Work out the finished part from the listing and answer in its coordinate system (mm). Face numbers are marked on the shaded views. A direction names the side the tool comes from. Coordinates: 2 decimals unless noted, no trailing zeros. Write each loop counter-clockwise with the first axis right and the second up, starting at its lowest first coordinate (ties: lowest second). Pieces come first, ordered by that corner, then holes. Notation, with made-up numbers: M -18,-19.5 L -7,-19.5 A13 ccw -7,-11.5 Z; hole C 70,28.5 d5. An arc over 180 degrees is marked long. Use CSV: the item, a comma, the result in double quotes.
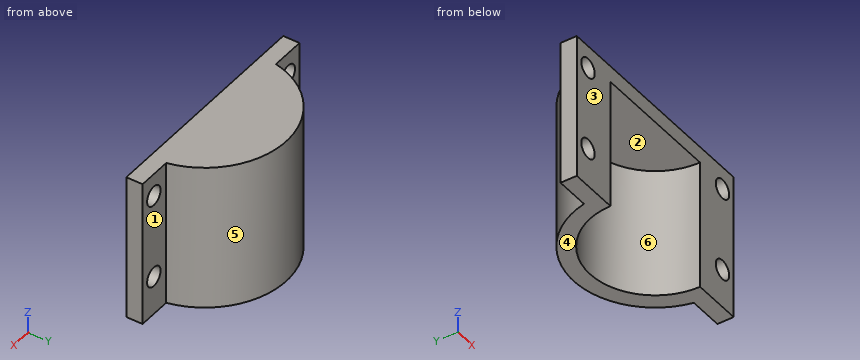
from build123d import *

# Parameters (mm, degrees)
SKETCH1_W                 = 70
SKETCH1_H                 = 50
BOSS_EXTRUDE1_DEPTH       = 30
CAVITY1_START             = -20
CAVITY1_DEPTH             = 40
CAVITY1_START_2           = -25
CAVITY1_2_DEPTH           = 5
CUT_EXTRUDE1_DEPTH        = 65.420493634
CUT_EXTRUDE1_DEPTH_BACK   = 65.420493634
F_6_0MM_DOWEL_HOLE1_D     = 6
F_6_0MM_DOWEL_HOLE1_DEPTH = 10
F_6_0MM_DOWEL_HOLE1_TIP   = 1.802581857
CUT_EXTRUDE3_DEPTH        = 5


# Read off the part's stored shape, not the designer's step: Cavity1
with BuildPart() as part:
    # Sketch1 → Boss-Extrude1 (new body)
    with BuildSketch(Plane(origin=(0, 0, 0), x_dir=(1, 0, 0), z_dir=(0, 1, 0))):
        Rectangle(SKETCH1_W, SKETCH1_H)
    extrude(amount=BOSS_EXTRUDE1_DEPTH)

    # Cavity1 outline → Cavity1 (cut)
    with BuildSketch(Plane.XY.offset(CAVITY1_START)):
        with BuildLine():
            ThreePointArc((20, 0), (0, 20), (-20, 0))
            Line((-20, 0), (20, 0))
        make_face()
    extrude(amount=CAVITY1_DEPTH, mode=Mode.SUBTRACT)

    # Cavity1 2 outline → Cavity1 2 (cut)
    with BuildSketch(Plane.XY.offset(CAVITY1_START_2)):
        with BuildLine():
            Line((-10, 0), (10, 0))
            ThreePointArc((10, 0), (0, 10), (-10, 0))
        make_face()
    extrude(amount=CAVITY1_2_DEPTH, mode=Mode.SUBTRACT)

    # Sketch2 → Cut-Extrude1 (cut, two sides: drawn at the far end of the back side and taken through both)
    with BuildSketch(Plane(origin=(0, 0, 20), x_dir=(-1, 0, 0), z_dir=(0, 0, -1)).offset(-CUT_EXTRUDE1_DEPTH_BACK)):
        with BuildLine():
            Line((-35, 30), (-35, 5))
            Line((-35, 5), (-24.494897428, 5))
            ThreePointArc((-24.494897428, 5), (0, 25), (24.494897428, 5))
            Line((24.494897428, 5), (35, 5))
            Line((35, 5), (35, 30))
            Line((35, 30), (-35, 30))
        make_face()
    extrude(amount=CUT_EXTRUDE1_DEPTH + CUT_EXTRUDE1_DEPTH_BACK, mode=Mode.SUBTRACT)

    # Ø6.0mm Dowel Hole1
    with Locations(Plane(origin=(0, 0, 0), x_dir=(-1, 0, 0), z_dir=(0, -1, 0))):
        with Locations((-30, 8), (-30, -18), (30, 8), (30, -18)):
            Hole(F_6_0MM_DOWEL_HOLE1_D / 2, depth=F_6_0MM_DOWEL_HOLE1_DEPTH)
            with Locations((0, 0, -(F_6_0MM_DOWEL_HOLE1_DEPTH + F_6_0MM_DOWEL_HOLE1_TIP / 2))):  # 118° drill point
                Cone(0, F_6_0MM_DOWEL_HOLE1_D / 2, F_6_0MM_DOWEL_HOLE1_TIP, mode=Mode.SUBTRACT)

    # Sketch6 → Cut-Extrude3 (cut)
    with BuildSketch(Plane(origin=(0, 0, -25), x_dir=(-1, 0, 0), z_dir=(0, 0, -1))):
        with BuildLine():
            Line((35, 5), (24.494897428, 5))
            ThreePointArc((24.494897428, 5), (0, 25), (-24.494897428, 5))
            Line((-24.494897428, 5), (-35, 5))
            Line((-35, 5), (-35, 0))
            Line((-35, 0), (-10, 0))
            ThreePointArc((-10, 0), (0, 10), (10, 0))
            Line((10, 0), (35, 0))
            Line((35, 0), (35, 5))
        make_face()
    extrude(amount=-CUT_EXTRUDE3_DEPTH, mode=Mode.SUBTRACT)


solid = part.part
Item 1: A tool of negligible diameter and unlimited length cuts with its end or side. For the marked faces 1, 2 and 3, from which of +Z, -Z, +X, -X, +Y, -Y can it reach the whole face along a straight path? Write none if from no direction.
Answer:
face 1,"+Z, -Z, +X, +Y"
face 2,"-Z, -Y"
face 3,"+Z, -Z, +X, -X, -Y"
Item 2: The part is cut by section A-A (x = -30). Write down the section's boundary in (y, z), then the cut area to 3 significant figures.
Answer:
outline,"M 0,-20 L 5,-20 L 5,-11 L 0,-11 Z; M 0,-5 L 5,-5 L 5,15 L 0,15 Z; M 0,21 L 5,21 L 5,25 L 0,25 Z"
area,"165 mm2"
Item 3: For a pull along X with two mould halves and no side action, classify the marked faces 4, 5 and 6 as released by +X, released by -X, zero draft, split by the parting line, or undercut.
Answer:
face 4,"zero draft"
face 5,"split by the parting line"
face 6,"undercut"
Item 4: Consider probe 1 along Z at (x, y) = (-30, 3.6); probe 2 along X at (y, z) = (2.5, 18); probe 3 along X at (y, z) = (3.25, 19.5). Determine where each line is inside the solid, lowest interval first.
Answer:
probe 1,"z = -20 to -11, -5 to 15, 21 to 25"
probe 2,"x = -35 to -33, -27 to -19.84, 19.84 to 27, 33 to 35"
probe 3,"x = -35 to -32.6, -27.4 to -19.73, 19.73 to 27.4, 32.6 to 35"
Item 5: The part is cut by section C-C (y = 2). Write down the section's boundary in (x, z), then the cut area to 3 significant figures.
Answer:
outline,"M -35,-20 L -19.9,-20 L -19.9,20 L 19.9,20 L 19.9,-20 L 35,-20 L 35,25 L -35,25 Z; hole C -30,-8 d6; hole C -30,18 d6; hole C 30,-8 d6; hole C 30,18 d6"
area,"1,440 mm2"
Item 6: The part is cut by section B-B (z = -8). Write down the section's boundary in (x, y).
Answer:
outline,"M -35,0 L -33,0 L -33,5 L -35,5 Z; M -27,0 L -20,0 A20 cw 20,0 L 27,0 L 27,5 L 24.49,5 A25 ccw -24.49,5 L -27,5 Z; M 33,0 L 35,0 L 35,5 L 33,5 Z"
Item 7: The part is cut by section D-D (z = 6.5). Write down the section's boundary in (x, y), then the cut area to 3 significant figures.
Answer:
outline,"M -35,0 L -20,0 A20 cw 20,0 L 35,0 L 35,5 L 24.49,5 A25 ccw -24.49,5 L -35,5 Z"
area,"455 mm2"
Item 8: Given pin 1 (3 mm diameter, centred on y = 15, z = 4.5, fed in from +X); pin 2 (8.5 mm diameter, centred on x = -29.5, z = 6, fed in from +Y); pin 3 (6 mm diameter, centred on y = 22, z = 4, fed in from +X); pin 4 (6 mm diameter, centred on x = 27.5, z = 13.5, fed in from -Y), each flat-ended and moving along its own axis, determine where each tip first touches the part or whether it passes through.
Answer:
pin 1,"stops at x = 21.04"
pin 2,"stops at y = 5"
pin 3,"stops at x = 16.25"
pin 4,"stops at y = 0"
